Geometry: final body of the model. Coordinates: model frame, mm. A direction names the side the tool comes from. Round coordinates to 2 decimals unless told otherwise and drop trailing zeros. Write each loop counter-clockwise with the first axis right and the second up, starting at its lowest first coordinate (ties: lowest second). Pieces come first, ordered by that corner, then holes. Notation, with made-up numbers: M -2.75,43 L 7.25,43 A7 cw 7.25,47 Z; hole C 1.5,16.25 d8. An arc over 180 degrees is marked long. Use one line per item in the form item = value. Start each with the question number.
Autodesk Inventor part; units mm, degrees
ref_plane "YZ Plane" through (0, 0, 0) normal (1, 0, 0) x (0, 1, 0)
ref_plane "XZ Plane" through (0, 0, 0) normal (0, 1, 0) x (-1, 0, 0)
ref_plane "XY Plane" through (0, 0, 0) normal (0, 0, 1) x (1, 0, 0)
sketch "Sketch1" plane through (0, 0, 0) normal (0, 0, 1) x (1, 0, 0)
  line L0 (0, 0) -> (0, 12)
  line L1 (0, 12) -> (-1.9, 12)
  line L2 (-1.9, 12) -> (-1.9, 10)
  line L3 (-1.9, 10) -> (-1, 10)
  line L4 (-1, 10) -> (-1, 0)
  line L5 (-1, 0) -> (0, 0)
  dimension "d0" = 10
  dimension "d1" = 2
  dimension "d2" = 1
  dimension "d3" = 1.9
revolve "Revolution1" add sketch "Sketch1" angle 360 about axis through (0, 0, 0) along (0, 1, 0)
sketch "Sketch2" plane through (0, 12, 0) normal (0, 1, 0) x (1, 0, 0)
  line L0 (-0.433, -0.75) -> (-0.866, 0)
  line L1 (-0.866, 0) -> (-0.433, 0.75)
  line L2 (-0.433, 0.75) -> (0.433, 0.75)
  line L3 (0.433, 0.75) -> (0.866, 0)
  line L4 (0.866, 0) -> (0.433, -0.75)
  line L5 (0.433, -0.75) -> (-0.433, -0.75)
  point P0 (0, 0)
  point P1 (0, 0)
  dimension "d5" = 1.5
extrude "Extrusion1" cut sketch "Sketch2" against normal blind 2
fillet "Fillet1" radius 0.3 6 edges at (0, 12, -0.75) (0.6495, 12, -0.375) (0.6495, 12, 0.375) (0, 12, 0.75) (-0.6495, 12, 0.375) (-0.6495, 12, -0.375)
fillet "Fillet2" radius 0.3 1 edges at (1.9, 12, 0)
thread "Thread1"
properties part number "Screw_StainlessSteal_M2_SocketCap_10mm" material "Stainless Steel"
1. Ray query, probe 1 along Z at (x, y) = (0.1, 10.75); probe 2 along Y at (x, z) = (-0.1, -1.15); probe 3 along X at (y, z) = (5.5, -0.05). Return the intervals inside material, ascending.
2. Set-up query: faces 4 (the face through (0, 11, 0.75)), 5 (the face through (0, 0, 0)). Return all of +Z, -Z, +X, -X, +Y, -Y with unobstructed straight access to the full face (end or side cutting, diameter ignored); none if empty.
3. Contact query for flat-ended pins moving along their axis: pin 1 (1.2 mm diameter, centred on x = -0.5, z = 0.5, fed in from +Y); pin 2 (1 mm diameter, centred on x = -0.5, y = 2.5, fed in from +Z). Output: stop coordinate, or through.
4. Pull-direction query (X, two-part tool) for faces 1 (the face through (0, 10, 0)), 2 (the face through (0, 5, 1)), 3 (the face through (-1, 10, -1)); classes: released by +X, released by -X, zero draft, split by the parting line, or undercut.
5. Section query A-A (x = 0). Return loops of the section in (y, z), then the cut area to 3 significant figures.
6. Section query B-B (y = 1). Return loops of the section in (x, z), then the cut area to 3 significant figures.
Checks:
q1.probe_1 = -1.9 to -0.75, 0.75 to 1.9
q1.probe_2 = 10 to 12
q1.probe_3 = -1 to 1
q2.face_4 = +Y
q2.face_5 = +Z, -Z, +X, -X, -Y
q3.pin_1 = 12
q3.pin_2 = 1
q4.face_1 = undercut
q4.face_2 = split by the parting line
q4.face_3 = zero draft
q5.outline = M 0,-1 L 10,-1 L 10,-1.9 L 11.7,-1.9 A0.3 ccw 12,-1.6 L 12,-1.05 A0.3 ccw 11.7,-0.75 L 10,-0.75 L 10,0.75 L 11.7,0.75 A0.3 ccw 12,1.05 L 12,1.6 A0.3 ccw 11.7,1.9 L 10,1.9 L 10,1 L 0,1 Z
q5.area = 24.5 mm^2
q6.outline = C 0,0 d2
q6.area = 3.14 mm^2
